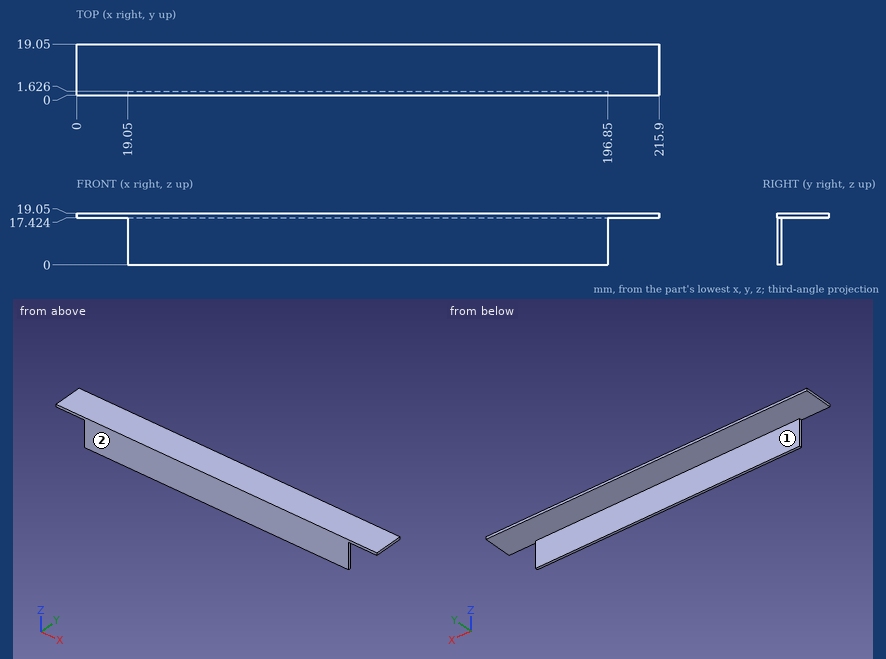
Source: three-view drawing plus pictorial views. Frame: mm from the lowest corner of the part. A direction names the side the tool comes from. Give positions to 0.01 mm unless a question says otherwise; leave off trailing zeros. Write each question's results on one line, items separated by ' | '. Start each with the question number.
Item 1: Line query: line 1 (Y direction, x = 44, z = 17.25) (1 decimal). Output: solid intervals per line, ascending.
Item 2: Set-up query: the marked faces 1 and 2. Return all of +Z, -Z, +X, -X, +Y, -Y with unobstructed straight access to the full face (end or side cutting, diameter ignored); none if empty.
Item 3: Contact query for flat-ended pins moving along their axis: P1, Ø10, axis at x = 154.5, y = 5, coming from the -Z side; P2, Ø8, axis at x = 110.5, y = 6.5, coming from the -Z side; P3, Ø1.3, axis at y = 1, z = 6.5, coming from the -X side; P4, Ø1, axis at x = 154.5, z = 9.5, coming from the +Y side. Output: stop coordinate, or through.
Established:
1) line 1: 0 to 1.6
2) face 1: -Z, +X, -X, +Y | face 2: +Z, -Z, +X, -X, -Y
3) P1: z = 0 | P2: z = 17.42 | P3: x = 19.05 | P4: y = 1.63
